from build123d import *

# Parameters (mm, degrees)
SKETCH1_W              = 76.2
SKETCH1_H              = 241.3
SKETCH1_W_2            = 63.5
SKETCH1_H_2            = 228.6
BOSS_EXTRUDE1_DEPTH    = 44.45
FILLET1_R              = 12.7
SKETCH2_W              = 76.2
SKETCH2_H              = 241.3
BOSS_EXTRUDE2_DEPTH    = 6.35
BOSS_EXTRUDE3_DEPTH    = 44.45
F_10_32_TAPPED_HOLE1_D = 4.0386
BOSS_EXTRUDE4_DEPTH    = 44.45


with BuildPart() as part:
    # Sketch1 → Boss-Extrude1 (new body)
    with BuildSketch(Plane.XY):
        with Locations((38.1, -120.65)):
            Rectangle(SKETCH1_W, SKETCH1_H)
        with Locations((38.1, -120.65)):
            Rectangle(SKETCH1_W_2, SKETCH1_H_2, mode=Mode.SUBTRACT)
    extrude(amount=BOSS_EXTRUDE1_DEPTH)

    # Fillet1
    fillet1_edges = [part.edges().sort_by_distance(p)[0] for p in [
        (6.35, -6.35, 22.225),
        (6.35, -234.95, 22.225),
        (69.85, -234.95, 22.225),
        (69.85, -6.35, 22.225),
    ]]
    fillet(fillet1_edges, radius=FILLET1_R)

    # Sketch2 → Boss-Extrude2 (add)
    with BuildSketch(Plane(origin=(0, 0, 0), x_dir=(-1, 0, 0), z_dir=(0, 0, -1))):
        with Locations((-38.1, -120.65)):
            Rectangle(SKETCH2_W, SKETCH2_H)
    extrude(amount=BOSS_EXTRUDE2_DEPTH)

    # Sketch3 → Boss-Extrude3 (add)
    with BuildSketch(Plane.XY.offset(44.45)):
        with BuildLine():
            Line((60.325, -120.65), (60.325, -133.35))
            ThreePointArc((60.325, -133.35), (67.204166667, -138.1125), (69.85, -146.05))
            Line((69.85, -146.05), (69.85, -107.95))
            ThreePointArc((69.85, -107.95), (67.204166667, -115.8875), (60.325, -120.65))
        make_face()
    boss_extrude3 = extrude(amount=-BOSS_EXTRUDE3_DEPTH)

    # Mirror1: Boss-Extrude3 across plane
    add(boss_extrude3.mirror(Plane.ZY.offset(-38.1)))

    # #10-32 Tapped Hole1 (through all)
    with Locations(Plane.XY.offset(44.45)):
        with Locations((4.7625, -4.7625), (71.4375, -4.7625), (71.4375, -127), (4.7625, -127), (4.7625, -236.5375), (71.4375, -236.5375)):
            Hole(F_10_32_TAPPED_HOLE1_D / 2)

    # Sketch8 → Boss-Extrude4 (add)
    with BuildSketch(Plane.XY.offset(44.45)):
        with BuildLine():
            Line((19.05, -209.55), (57.15, -209.55))
            ThreePointArc((57.15, -209.55), (66.130256121, -213.269743879), (69.85, -222.25))
            Line((69.85, -222.25), (69.85, -190.5))
            ThreePointArc((69.85, -190.5), (66.130256121, -199.480256121), (57.15, -203.2))
            Line((57.15, -203.2), (19.05, -203.2))
            ThreePointArc((19.05, -203.2), (10.069743879, -199.480256121), (6.35, -190.5))
            Line((6.35, -190.5), (6.35, -222.25))
            ThreePointArc((6.35, -222.25), (10.069743879, -213.269743879), (19.05, -209.55))
        make_face()
    extrude(amount=-BOSS_EXTRUDE4_DEPTH)


solid = part.part
Verification items for the finished model (mm, model axes). A direction names the side the tool comes from. Coordinates: 2 decimals unless noted, no trailing zeros. Order: outer loops, then holes, each group sorted by start corner. A loop starts at its lowest first (then second) coordinate and runs counter-clockwise, first axis right, second up.
Item 1: Release check for a two-part mould opening along Y. For faces 3 (the face through (39, -241.3, 19)), 4 (the face through (39, -119, -6.35)), 5 (the face through (67.132, -138.017, 22.536)) record: +Y half, -Y half, draft (parallel to the pull), parting line (faces both ways), or undercut.
Filled in:
face 3: -Y half
face 4: draft
face 5: undercut
Item 2: Depth check by flat-ended pin: pin 1 (3 mm diameter, centred on x = 50.5, y = -69, fed in from +Z); pin 2 (2.5 mm diameter, centred on x = 4.76, y = -236.54, fed in from +Z). Enter the tip coordinate at first touch or a pass-through.
Filled in:
pin 1: stops at z = 0
pin 2: passes through
Item 3: Access from +Z, -Z, +X, -X, +Y, -Y to the whole of each face (thin tool, end or side, straight path). Record for faces 1 (the face through (5.2, -128.97, 18.69)), 2 (the face through (67.275, -115.792, 22.536)).
Filled in:
face 1: +Z, -Z
face 2: +Z
Item 4: Section check A-A, the plane y = -149. Enter the section's corners in (x, z).
Filled in:
outline: (0, -6.35) - (76.2, -6.35) - (76.2, 44.45) - (69.85, 44.45) - (69.85, 0) - (6.35, 0) - (6.35, 44.45) - (0, 44.45) - close
Item 5: Section check C-C, the plane z = 25. Give the number of separate pieces and of enclosed holes in the cut face, then the cut area to 3 significant figures.
Filled in:
separate pieces: 1
enclosed holes: 8
area: 4,840 mm2
Item 6: Material ranges on L1, parallel to Y at x = 25, z = 17.5; L2, parallel to X at y = -91.5, z = 16.5, recorded low to high.
Filled in:
L1: y = -241.3 to -234.95, -209.55 to -203.2, -6.35 to 0
L2: x = 0 to 6.35, 69.85 to 76.2
Item 7: Section check B-B, the plane x = 40. Enter the section's corners in (y, z).
Filled in:
outline: (-241.3, -6.35) - (0, -6.35) - (0, 44.45) - (-6.35, 44.45) - (-6.35, 0) - (-203.2, 0) - (-203.2, 44.45) - (-209.55, 44.45) - (-209.55, 0) - (-234.95, 0) - (-234.95, 44.45) - (-241.3, 44.45) - close
Item 8: Section check D-D, the plane x = 10. Enter the section's corners in (y, z), then the cut area to 3 significant figures.
Filled in:
outline: (-241.3, -6.35) - (0, -6.35) - (0, 44.45) - (-10.14, 44.45) - (-10.14, 0) - (-117.07, 0) - (-117.07, 44.45) - (-136.93, 44.45) - (-136.93, 0) - (-199.41, 0) - (-199.41, 44.45) - (-213.34, 44.45) - (-213.34, 0) - (-231.16, 0) - (-231.16, 44.45) - (-241.3, 44.45) - close
area: 3,940 mm2
